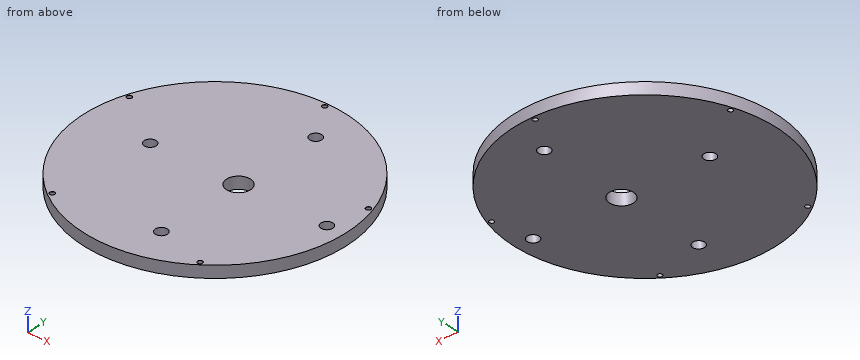
```python
from build123d import *

# Parameters (mm, degrees)
SKETCH1_R                       = 27.5
BOSS_EXTRUDE1_DEPTH             = 1.25
SKETCH3_R                       = 2.5
SKETCH3_R_2                     = 1.25
CUT_EXTRUDE1_DEPTH              = 1
CUT_EXTRUDE1_DEPTH_BACK         = 3.5
F_1_0MM_DOWEL_HOLE1_D           = 1
F_1_0MM_DOWEL_HOLE1_CSINK_D     = 1.05
F_1_0MM_DOWEL_HOLE1_CSINK_ANGLE = 90
CIRPATTERN1_COUNT               = 5


with BuildPart() as part:
    # Sketch1 → Boss-Extrude1 (new body, symmetric)
    with BuildSketch(Plane.XY):
        Circle(SKETCH1_R)
    extrude(amount=BOSS_EXTRUDE1_DEPTH, both=True)

    # Sketch3 → Cut-Extrude1 (cut, two sides)
    with BuildSketch(Plane.XY.offset(1.25)) as cut_extrude1_sk:
        with Locations((5, 0)):
            Circle(SKETCH3_R)
        with Locations((5, 18.75)):
            Circle(SKETCH3_R_2)
        with Locations((-13.75, 0)):
            Circle(SKETCH3_R_2)
        with Locations((23.75, 0)):
            Circle(SKETCH3_R_2)
        with Locations((5, -18.75)):
            Circle(SKETCH3_R_2)
    extrude(amount=CUT_EXTRUDE1_DEPTH, mode=Mode.SUBTRACT)
    extrude(cut_extrude1_sk.sketch, amount=-CUT_EXTRUDE1_DEPTH_BACK, mode=Mode.SUBTRACT)

    # Ø1.0mm Dowel Hole1 (through all)
    with Locations(Plane(origin=(0, 26.666666667, 1.25), x_dir=(1, 0, 0), z_dir=(0, 0, 1))):
        with Locations((0, 0)):
            f_1_0mm_dowel_hole1 = CounterSinkHole(F_1_0MM_DOWEL_HOLE1_D / 2, F_1_0MM_DOWEL_HOLE1_CSINK_D / 2, counter_sink_angle=F_1_0MM_DOWEL_HOLE1_CSINK_ANGLE)

    # CirPattern1: Ø1.0mm Dowel Hole1 ×5 about axis
    cirpattern1_axis = Axis((0, 0, 0), (0, 0, 1))
    for i in range(1, CIRPATTERN1_COUNT):
        add(f_1_0mm_dowel_hole1.rotate(cirpattern1_axis, i * 360 / CIRPATTERN1_COUNT), mode=Mode.SUBTRACT)


solid = part.part
```
For this review, take the finished solid that the model builds, in its own axes (mm). Give positions to 0.01 mm unless a question says otherwise; leave off trailing zeros. Write each loop counter-clockwise with the first axis right and the second up, starting at its lowest first coordinate (ties: lowest second). Pieces come first, ordered by that corner, then holes.
Item 1: Take a section at D-D (z = -0.4). Give the number of separate pieces and of enclosed holes in the cut face, and give its area (3 significant figures).
Item 2: Take a section at C-C (y = 18.75). Give the boundary of the cut face in (x, z).
Item 3: Wall thickness on probe 1 along Y at (x, z) = (5, 0.75); probe 2 along Y at (x, z) = (-13, 0); probe 3 along Y at (x, z) = (-13.75, -0.2): over which ranges is each line inside the solid? List them lowest first.
Item 4: Take a section at B-B (x = -13.75). Give the boundary of the cut face in (y, z), and give its area (3 significant figures).
Item 5: Insertion check: P1, Ø1, axis at y = -7.5, z = 1, coming from the +X side. The pin has a flat end and moves straight along its axis. Give the tip position at first contact, or say it passes through.
Item 6: Take a section at A-A (y = 0). Give the boundary of the cut face in (x, z).
Established:
1. separate pieces: 1
1. enclosed holes: 10
1. area: 2,330 mm2
2. outline: (-20.12, -1.25) - (3.75, -1.25) - (3.75, 1.25) - (-20.12, 1.25) - close; (6.25, -1.25) - (20.12, -1.25) - (20.12, 1.25) - (6.25, 1.25) - close
3. probe 1: y = -27.04 to -20, -17.5 to -2.5, 2.5 to 17.5, 20 to 27.04
3. probe 2: y = -24.23 to -1, 1 to 24.23
3. probe 3: y = -23.82 to -1.25, 1.25 to 23.82
4. outline: (-23.82, -1.25) - (-1.25, -1.25) - (-1.25, 1.25) - (-23.82, 1.25) - close; (1.25, -1.25) - (23.82, -1.25) - (23.82, 1.25) - (1.25, 1.25) - close
4. area: 113 mm2
5. P1: stops at x = 26.59
6. outline: (-27.5, -1.25) - (-15, -1.25) - (-15, 1.25) - (-27.5, 1.25) - close; (-12.5, -1.25) - (2.5, -1.25) - (2.5, 1.25) - (-12.5, 1.25) - close; (7.5, -1.25) - (22.5, -1.25) - (22.5, 1.25) - (7.5, 1.25) - close; (25, -1.25) - (27.5, -1.25) - (27.5, 1.25) - (25, 1.25) - close
